from build123d import *

# Parameters (mm, degrees)
SKETCH1_W           = 200
SKETCH1_H           = 170
BOSS_EXTRUDE1_DEPTH = 3
SKETCH2_W           = 24.321835298
SKETCH2_H           = 70
CUT_EXTRUDE1_DEPTH  = 100
SKETCH3_R           = 1.5
CUT_EXTRUDE2_DEPTH  = 100
SKETCH4_R           = 1.5
CUT_EXTRUDE3_DEPTH  = 100
FILLET1_R           = 30


with BuildPart() as part:
    # Sketch1 → Boss-Extrude1 (new body)
    with BuildSketch(Plane(origin=(0, 0, 0), x_dir=(1, 0, 0), z_dir=(0, 1, 0))):
        Rectangle(SKETCH1_W, SKETCH1_H)
    extrude(amount=BOSS_EXTRUDE1_DEPTH)

    # Sketch2 → Cut-Extrude1 (cut)
    with BuildSketch(Plane(origin=(0, 3, 0), x_dir=(1, 0, 0), z_dir=(0, 1, 0))):
        with Locations((-62.239691906, 0)):
            Rectangle(SKETCH2_W, SKETCH2_H)
    extrude(amount=-CUT_EXTRUDE1_DEPTH, mode=Mode.SUBTRACT)

    # Sketch3 → Cut-Extrude2 (cut)
    with BuildSketch(Plane(origin=(0, 3, 0), x_dir=(1, 0, 0), z_dir=(0, 1, 0))):
        with Locations((-78.38, -71.5)):
            Circle(SKETCH3_R)
        with Locations((-78.38, 71.5)):
            Circle(SKETCH3_R)
        with Locations((78.38, 71.5)):
            Circle(SKETCH3_R)
        with Locations((78.38, -71.5)):
            Circle(SKETCH3_R)
    extrude(amount=-CUT_EXTRUDE2_DEPTH, mode=Mode.SUBTRACT)

    # Sketch4 → Cut-Extrude3 (cut)
    with BuildSketch(Plane(origin=(0, 3, 0), x_dir=(1, 0, 0), z_dir=(0, 1, 0))):
        with Locations((-14.58, -81)):
            Circle(SKETCH4_R)
        with Locations((14.58, -81)):
            Circle(SKETCH4_R)
        with Locations((-14.58, -70)):
            Circle(SKETCH4_R)
        with Locations((14.58, -70)):
            Circle(SKETCH4_R)
        with Locations((-14.58, 81)):
            Circle(SKETCH4_R)
        with Locations((-14.58, 70)):
            Circle(SKETCH4_R)
        with Locations((14.58, 81)):
            Circle(SKETCH4_R)
        with Locations((14.58, 70)):
            Circle(SKETCH4_R)
    extrude(amount=-CUT_EXTRUDE3_DEPTH, mode=Mode.SUBTRACT)

    # Fillet1
    fillet1_edges = [part.edges().sort_by_distance(p)[0] for p in [
        (100, 1.5, 85),
        (-100, 1.5, 85),
        (-100, 1.5, -85),
        (100, 1.5, -85),
    ]]
    fillet(fillet1_edges, radius=FILLET1_R)


solid = part.part
Work out the finished part from the listing and answer in its coordinate system (mm). Coordinates: 2 decimals unless noted, no trailing zeros. Loops run counter-clockwise (first coordinate to the right, second up) from the corner with the lowest first, then second, coordinate; pieces in that order, holes last. Notation, with made-up numbers: (-1.5, 6) -> (31.5, 6) arc R18 ccw to (31.5, 39) -> close; hole circle Ø5 at (79.25, 53.5). An arc over 180 degrees is marked (long way). Write each question's results on one line, items separated by ' | '. Start each with the question number.
1) Consider line 1 along X through (y, z) = (0.9, 81); line 2 along Z through (x, y) = (-14.58, 1.95); line 3 along X through (y, z) = (0.85, -4.5). Determine where each line is inside the solid, lowest interval first.
2) Find section B-B on y = 0.65. Count the separate pieces of the cut face and the enclosed holes in it, then the cut area to 3 significant figures.
3) Find section A-A on z = 5. Determine the outline of the cut face in (x, y).
Response values:
1) line 1: x = -84.97 to -16.08, -13.08 to 13.08, 16.08 to 84.97 | line 2: z = -85 to -82.5, -79.5 to -71.5, -68.5 to 68.5, 71.5 to 79.5, 82.5 to 85 | line 3: x = -100 to -74.4, -50.08 to 100
2) separate pieces: 1 | enclosed holes: 13 | area: 31,400 mm^2
3) outline: (-100, 0) -> (-74.4, 0) -> (-74.4, 3) -> (-100, 3) -> close; (-50.08, 0) -> (100, 0) -> (100, 3) -> (-50.08, 3) -> close
